Geometry check sheet. Reference: the model listing, model coordinates, mm. Face numbers are marked on the shaded views. A direction names the side the tool comes from. Coordinates: 2 decimals unless noted, no trailing zeros. Write each loop counter-clockwise with the first axis right and the second up, starting at its lowest first coordinate (ties: lowest second). Pieces come first, ordered by that corner, then holes. Notation, with made-up numbers: (-32.75, -4) - (-27.75, -4) arc R12 ccw to (-27.75, 7) - close; hole circle Ø7 at (81, 86.5). An arc over 180 degrees is marked (long way). Answer as a JSON object with one key per item and string values. Group by question number.
from build123d import *

# Parameters (mm, degrees)
F1_DEPTH        = 25
F3_R            = 15
F4_DEPTH        = 52
F6_D            = 13.2
F6_CBORE_D      = 19.25
F6_CBORE_DEPTH  = 0
F8_D            = 13.2
F8_CBORE_D      = 19.25
F8_CBORE_DEPTH  = 0
F10_D           = 13.2
F10_CBORE_D     = 19.25
F10_CBORE_DEPTH = 0
F11_W           = 35.8968544751
F11_H           = 52.9583077878
F12_DEPTH       = 58


with BuildPart() as f1:
    # F0 (on Front) → F1 (new body)
    with BuildSketch(Plane.XZ):
        with BuildLine():
            Line((-25, -40), (25, -40))
            Line((25, -40), (25, 40))
            ThreePointArc((25, 40), (10.5, 25.5), (-4, 40))
            Line((-4, 40), (-25, 40))
            Line((-25, 40), (-25, -40))
        make_face()
        with BuildLine():
            ThreePointArc((-4, 40), (10.5, 25.5), (25, 40))
            Line((25, 40), (-4, 40))
        make_face()
        with BuildLine():
            Line((-4, 40), (25, 40))
            ThreePointArc((25, 40), (10.5, 54.5), (-4, 40))
        make_face()
    extrude(amount=F1_DEPTH)

    # F3 (on face) → F4 (join)
    with BuildSketch(Plane(origin=(0, 17.3205080757, -10), x_dir=(1, 0, 0), z_dir=(0, -0.8660254038, 0.5))):
        with Locations((25, -34.6410161514)):
            Circle(F3_R)
    extrude(amount=F4_DEPTH)

    # F6 (through all)
    with Locations(Plane(origin=(0, 17.3205080757, -10), x_dir=(-1, 0, 0), z_dir=(0, 0.8660254038, -0.5))):
        with Locations((-25, -34.6410161514)):
            CounterBoreHole(F6_D / 2, F6_CBORE_D / 2, F6_CBORE_DEPTH)

    # F8 (through all)
    with Locations(Plane(origin=(0, 0, 0), x_dir=(-1, 0, 0), z_dir=(0, 1, 0))):
        with Locations((-10.5, 40)):
            CounterBoreHole(F8_D / 2, F8_CBORE_D / 2, F8_CBORE_DEPTH)

    # F10 (through all)
    with Locations(Plane.XY.offset(40)):
        with Locations((-14.5, -12.5)):
            CounterBoreHole(F10_D / 2, F10_CBORE_D / 2, F10_CBORE_DEPTH)

    # F11 (on Right) → F12 (cut)
    with BuildSketch(Plane.YZ):
        with Locations((-42.9484272376, -22.4903533235)):
            Rectangle(F11_W, F11_H)
    extrude(amount=F12_DEPTH, mode=Mode.SUBTRACT)


solid = f1.part
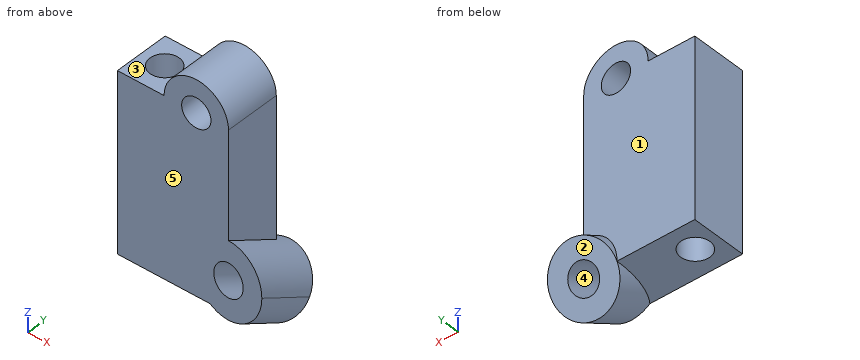
(1) Section check B-B (z = 10). Record the cut outline in (x, y).
(2) Draft check along Y on the marked faces 3, 4 and 5. Enter one of: +Y half, -Y half, draft (parallel to the pull), parting line (faces both ways), or undercut.
(3) Section check C-C (y = -14). Count the separate pieces of the cut face and the enclosed holes in it, and give its area (3 significant figures).
(4) Material ranges on L1, parallel to Z at x = 10.5, y = -8.5; L2, parallel to Y at x = -14, z = 23; L3, parallel to X at y = -8.5, z = -29, recorded low to high. Write a range as [from, to].
(5) Section check D-D (x = 29.5). Record the cut outline in (y, z).
(6) Section check A-A (x = -14.5). Record the cut outline in (y, z).
(7) Set-up check for the marked faces 1 and 2: record each of +Z, -Z, +X, -X, +Y, -Y from which the full face is reachable in a straight line by a thin tool's end or side.
(8) Gauge pin test, flat ends, axial feed: pin 1 (12.5 mm diameter, centred on y = -16.5, z = 4, fed in from +X); pin 2 (10 mm diameter, centred on x = -6, z = -30.5, fed in from +Y); pin 3 (15 mm diameter, centred on x = -14.5, y = -12.5, fed in from +Z). Record the tip position at first contact, or that the pin passes through.
Conclusion:
{
 "1": {"outline": "(-25, -25) - (25, -25) - (25, 0) - (-25, 0) - close; hole circle Ø13.2 at (-14.5, -12.5)"},
 "2": {"face 3": "draft", "face 4": "undercut", "face 5": "-Y half"},
 "3": {"separate pieces": "2", "enclosed holes": "2", "area": "3,500 mm^2"},
 "4": {"L1": "z = [-40, 33.4], [46.6, 54.5]", "L2": "y = [-25, -19.08], [-5.92, 0]", "L3": "x = [-25, -19.75], [-9.25, 21.04], [28.96, 39.04]"},
 "5": {"outline": "(-25, -42.09) - (-7.15, -52.39) - (-2.41, -44.18) - (-25, -31.14) - close; (-25, -19.99) - (2.41, -35.82) - (7.15, -27.61) - (-25, -9.04) - close"},
 "6": {"outline": "(-25, -40) - (-19.1, -40) - (-19.1, 40) - (-25, 40) - close; (-5.9, -40) - (0, -40) - (0, 40) - (-5.9, 40) - close"},
 "7": {"face 1": "+Z, -X, +Y", "face 2": "-Z, +X, -X, +Y"},
 "8": {"pin 1": "stops at x = 25", "pin 2": "stops at y = 0", "pin 3": "stops at z = 40"}
}
